from build123d import *

# Parameters (mm, degrees)
BOSS_EXTRUDE1_DEPTH                   = 4.7625
F_10_CLEARANCE_HOLE1_AT_2_COUNT       = 2
F_10_CLEARANCE_HOLE1_AT_2_PITCH       = 39.612434438
F_10_CLEARANCE_HOLE1_AT_3_COUNT       = 2
F_10_CLEARANCE_HOLE1_AT_3_PITCH       = 22.428811893
FILLET1_R                             = 2.54
F_52_0_0635_DIAMETER_HOLE1_AT_2_COUNT = 2
F_52_0_0635_DIAMETER_HOLE1_AT_2_PITCH = 14
F_52_0_0635_DIAMETER_HOLE1_AT_3_COUNT = 2
F_52_0_0635_DIAMETER_HOLE1_AT_3_PITCH = 16.124515497
F_52_0_0635_DIAMETER_HOLE1_AT_4_COUNT = 2
F_52_0_0635_DIAMETER_HOLE1_AT_4_PITCH = 8
CHAMFER4_SIZE                         = 0.762


with BuildPart() as part:
    # Sketch2 → Boss-Extrude1 (new body)
    with BuildSketch(Plane.XY.offset(49.981386822)):
        with BuildLine():
            Line((-91.534347313, -223.683915635), (-71.534347313, -223.683915635))
            Line((-71.534347313, -223.683915635), (-71.534347313, -209.683915635))
            Line((-71.534347313, -209.683915635), (-81.955963126, -191.43064496))
            ThreePointArc((-81.955963126, -191.43064496), (-86.661422004, -188.280866285), (-92.010183842, -190.139143919))
            Line((-92.010183842, -190.139143919), (-108.307938293, -206.803069118))
            ThreePointArc((-108.307938293, -206.803069118), (-109.919716645, -209.667777106), (-109.883203649, -212.954576174))
            Line((-109.883203649, -212.954576174), (-103.837901654, -234.553324441))
            ThreePointArc((-103.837901654, -234.553324441), (-97.573904916, -239.190042315), (-91.534347313, -234.264542164))
            Line((-91.534347313, -234.264542164), (-91.534347313, -223.683915635))
        make_face()
    extrude(amount=BOSS_EXTRUDE1_DEPTH)

    # Sketch7 → #10 Clearance Hole1 (revolve, cut)
    with BuildSketch(Plane(origin=(-97.722907594, -232.841790729, 54.743886822), x_dir=(0, -1, 0), z_dir=(1, 0, 0))):
        Polygon((0, 0), (0, 4.7625), (3.1877, 4.7625), (2.5527, 4.1275), (2.5527, 0.635), (3.1877, 0), align=None)
    f_10_clearance_hole1 = revolve(axis=Axis((-97.722907594, -232.841790729, 61.093886822), (0, 0, -1)), mode=Mode.SUBTRACT)

    # #10 Clearance Hole1 at 2: #10 Clearance Hole1 ×2
    with Locations(*[Vector(0.25881904510252135, 0.9659258262890682, 0) * (i * F_10_CLEARANCE_HOLE1_AT_2_PITCH) for i in range(1, F_10_CLEARANCE_HOLE1_AT_2_COUNT)]):
        add(f_10_clearance_hole1, mode=Mode.SUBTRACT)

    # #10 Clearance Hole1 at 3: #10 Clearance Hole1 ×2
    with Locations(*[Vector(-0.2695328680059712, 0.9629911905435459, 0) * (i * F_10_CLEARANCE_HOLE1_AT_3_PITCH) for i in range(1, F_10_CLEARANCE_HOLE1_AT_3_COUNT)]):
        add(f_10_clearance_hole1, mode=Mode.SUBTRACT)

    # Fillet1
    fillet1_edges = [part.edges().sort_by_distance(p)[0] for p in [
        (-71.534347313, -209.683915635, 52.362636822),
        (-71.534347313, -223.683915635, 52.362636822),
        (-91.534347313, -223.683915635, 52.362636822),
    ]]
    fillet(fillet1_edges, radius=FILLET1_R)

    # Sketch9 → #52 (0.0635) Diameter Hole1 (revolve, cut)
    with BuildSketch(Plane(origin=(-88.534347313, -212.683915635, 54.743886822), x_dir=(0, -1, 0), z_dir=(1, 0, 0))):
        Polygon((0, 0), (0, 4.7625), (1.44145, 4.7625), (0.80645, 4.1275), (0.80645, 0.635), (1.44145, 0), align=None)
    f_52_0_0635_diameter_hole1 = revolve(axis=Axis((-88.534347313, -212.683915635, 61.093886822), (0, 0, -1)), mode=Mode.SUBTRACT)

    # #52 (0.0635) Diameter Hole1 at 2: #52 (0.0635) Diameter Hole1 ×2
    with Locations(*[(i * F_52_0_0635_DIAMETER_HOLE1_AT_2_PITCH, 0, 0) for i in range(1, F_52_0_0635_DIAMETER_HOLE1_AT_2_COUNT)]):
        add(f_52_0_0635_diameter_hole1, mode=Mode.SUBTRACT)

    # #52 (0.0635) Diameter Hole1 at 3: #52 (0.0635) Diameter Hole1 ×2
    with Locations(*[Vector(0.86824314212446, -0.49613893835683254, 0) * (i * F_52_0_0635_DIAMETER_HOLE1_AT_3_PITCH) for i in range(1, F_52_0_0635_DIAMETER_HOLE1_AT_3_COUNT)]):
        add(f_52_0_0635_diameter_hole1, mode=Mode.SUBTRACT)

    # #52 (0.0635) Diameter Hole1 at 4: #52 (0.0635) Diameter Hole1 ×2
    with Locations(*[(0, -i * F_52_0_0635_DIAMETER_HOLE1_AT_4_PITCH, 0) for i in range(1, F_52_0_0635_DIAMETER_HOLE1_AT_4_COUNT)]):
        add(f_52_0_0635_diameter_hole1, mode=Mode.SUBTRACT)

    # Chamfer4
    chamfer4_edges = [part.edges().sort_by_distance(p)[0] for p in [
        (-97.573904916, -239.190042315, 49.981386822),
        (-106.860552651, -223.753950307, 49.981386822),
        (-109.919716645, -209.667777106, 49.981386822),
        (-100.159061068, -198.471106519, 49.981386822),
        (-86.661422004, -188.280866285, 49.981386822),
        (-86.661422004, -188.280866285, 54.743886822),
        (-100.159061068, -198.471106519, 54.743886822),
        (-109.919716645, -209.667777106, 54.743886822),
        (-106.860552651, -223.753950307, 54.743886822),
        (-97.573904916, -239.190042315, 54.743886822),
        (-76.912256817, -200.264604887, 49.981386822),
        (-76.912256817, -200.264604887, 54.743886822),
        (-91.534347313, -230.2442289, 49.981386822),
        (-71.534347313, -215.750934685, 49.981386822),
        (-81.534347313, -223.683915635, 49.981386822),
        (-72.278296088, -222.939966859, 49.981386822),
        (-71.619319422, -209.706464627, 49.981386822),
        (-71.534347313, -215.750934685, 54.743886822),
        (-91.534347313, -230.2442289, 54.743886822),
        (-81.534347313, -223.683915635, 54.743886822),
        (-72.278296088, -222.939966859, 54.743886822),
        (-71.619319422, -209.706464627, 54.743886822),
        (-90.790398537, -224.427864411, 49.981386822),
        (-90.790398537, -224.427864411, 54.743886822),
    ]]
    chamfer(chamfer4_edges, length=CHAMFER4_SIZE)


solid = part.part
Input: part model. Units: mm. Frame: model coordinates. Coordinates: 2 decimals unless noted, no trailing zeros. Write each loop counter-clockwise with the first axis right and the second up, starting at its lowest first coordinate (ties: lowest second). Pieces come first, ordered by that corner, then holes. Notation, with made-up numbers: M 67,41 L 97,41 A18 ccw 97,71 Z; hole C 17.25,-4 d8. An arc over 180 degrees is marked long. Answer as a JSON object with one key per item and string values. Group by question number.
(1) Section C-C on z = 51.5. Output: boundary loops of the cut face in (x, y), plus the area to 3 significant figures.
(2) Section A-A on x = -77. Output: boundary loops of the cut face in (y, z), plus the area to 3 significant figures.
(3) Mould query, pull axis X, two halves, no side actions, for faces 1 (the face through (-86.67, -188.92, 50.11)), 2 (the face through (-102.79, -213.6, 52.39)), 3 (the face through (-72.62, -222.63, 50.28)), 4 (the face through (-106.903, -223.603, 52.34)). Classes: pulls with the +X half, pulls with the -X half, needs draft (parallel to the pull), parting line crosses it, or undercut.
(4) Ray query, line 1 along X through (y, z) = (-212, 51.25); line 2 along Y through (x, z) = (-74.5, 53.15); line 3 along Y through (x, z) = (-89, 50.5). Return the intervals inside material, ascending. Write a range as [from, to].
(5) Contact query for flat-ended pins moving along their axis: P1, Ø2, axis at x = -74.53, y = -212.68, coming from the -Z side; P2, Ø2, axis at x = -88.53, y = -220.68, coming from the +Z side; P3, Ø2.5, axis at x = -74.53, y = -220.68, coming from the +Z side. Output: stop coordinate, or through.
(6) Section B-B on y = -216. Output: boundary loops of the cut face in (x, z), plus the area to 3 significant figures.
Result set:
{
 "1": {"outline": "M -109.88,-212.95 L -103.84,-234.55 A6.35 ccw -91.53,-234.26 L -91.53,-226.22 A2.54 cw -88.99,-223.68 L -74.07,-223.68 A2.54 ccw -71.53,-221.14 L -71.53,-210.36 A2.54 ccw -71.87,-209.1 L -81.96,-191.43 A6.35 ccw -92.01,-190.14 L -108.31,-206.8 A6.35 ccw Z; hole C -103.77,-211.24 d5.11; hole C -97.72,-232.84 d5.11; hole C -87.47,-194.58 d5.11; hole C -88.53,-220.68 d1.61; hole C -88.53,-212.68 d1.61; hole C -74.53,-220.68 d1.61; hole C -74.53,-212.68 d1.61", "area": "1,130 mm2"},
 "2": {"outline": "M -223.68,50.74 L -222.92,49.98 L -201.65,49.98 L -200.11,50.74 L -200.11,53.98 L -201.65,54.74 L -222.92,54.74 L -223.68,53.98 Z", "area": "111 mm2"},
 "3": {"face 1": "parting line crosses it", "face 2": "undercut", "face 3": "pulls with the +X half", "face 4": "pulls with the -X half"},
 "4": {"line 1": "x = [-110.07, -106.21], [-101.33, -88.96], [-88.11, -74.96], [-74.11, -71.53]", "line 2": "y = [-223.68, -221.49], [-219.88, -213.49], [-211.88, -204.49]", "line 3": "y = [-223.44, -221.48], [-219.89, -213.48], [-211.89, -196.77], [-192.39, -188.67]"},
 "5": {"P1": "stops at z = 50.42", "P2": "stops at z = 54.31", "P3": "stops at z = 54.56"},
 "6": {"outline": "M -109.03,50.74 L -108.24,49.98 L -72.3,49.98 L -71.53,50.74 L -71.53,53.98 L -72.3,54.74 L -108.24,54.74 L -109.03,53.98 Z", "area": "177 mm2"}
}
